```python
from build123d import *

# Parameters (mm, degrees)
RESSALTO_EXTRUS_O1_DEPTH = 0.3


with BuildPart() as part:
    # Esboço1 → Ressalto-extrusão1 (new body, symmetric)
    with BuildSketch(Plane.XY):
        with BuildLine():
            Line((17.891752756, 0.197947805), (17.891752756, -0.002052195))
            Line((17.891752756, -0.002052195), (17.091752756, -0.002052195))
            ThreePointArc((17.091752756, -0.002052195), (16.996884427, 0.013342816), (16.911752756, 0.057947805))
            Line((16.911752756, 0.057947805), (16.038199366, 0.968756691))
            ThreePointArc((16.038199366, 0.968756691), (16.005773821, 0.990473944), (15.967488688, 0.99804386))
            Line((15.967488688, 0.99804386), (12.407488688, 0.99))
            Line((12.407488688, 0.99), (10.557971552, 1.813458083))
            ThreePointArc((10.557971552, 1.813458083), (10.373577052, 1.832838725), (10.213007112, 1.740133627))
            Line((10.213007112, 1.740133627), (9.099531826, 0.503494039))
            Line((9.099531826, 0.503494039), (8.95090286, 0.637320161))
            Line((8.95090286, 0.637320161), (10.064378147, 1.873959748))
            ThreePointArc((10.064378147, 1.873959748), (10.331994714, 2.028468246), (10.639318881, 1.996167174))
            Line((10.639318881, 1.996167174), (12.45, 1.19))
            Line((12.45, 1.19), (15.967488688, 1.197947805))
            ThreePointArc((15.967488688, 1.197947805), (16.082345327, 1.175236263), (16.179620722, 1.11007984))
            Line((16.179620722, 1.11007984), (17.029007121, 0.256846352))
            ThreePointArc((17.029007121, 0.256846352), (17.094002269, 0.213258484), (17.170747658, 0.197947805))
            Line((17.170747658, 0.197947805), (17.891752756, 0.197947805))
        make_face()
    extrude(amount=RESSALTO_EXTRUS_O1_DEPTH, both=True)


solid = part.part
```
Source: CAD feature listing. Evaluate the final solid. Frame: model axes, mm. Give positions to 0.01 mm unless a question says otherwise; leave off trailing zeros. Loops run counter-clockwise (first coordinate to the right, second up) from the corner with the lowest first, then second, coordinate; pieces in that order, holes last. Notation, with made-up numbers: M -11.75,-12 L 21.25,-12 A27 cw 21.25,15 Z; hole C -9.75,-1.75 d1. An arc over 180 degrees is marked long. Put each result on its own line as item: value.
Q1. Line query: probe 1 along Y at (x, z) = (17.25, 0); probe 2 along Y at (x, z) = (15.5, -0.15); probe 3 along X at (y, z) = (0.95, -0.05). Output: solid intervals per line, ascending. Write a range as [from, to].
Response values:
probe 1: y = [0, 0.2]
probe 2: y = [1, 1.2]
probe 3: x = [9.23, 9.5], [16.06, 16.34]
Q2. Section C-C (y = 0.8). Return the cut outline in (x, z).
Response values:
outline: M 9.1,-0.3 L 9.37,-0.3 L 9.37,0.3 L 9.1,0.3 Z; M 16.2,-0.3 L 16.49,-0.3 L 16.49,0.3 L 16.2,0.3 Z
Q3. Pin query (flat end, axial travel): P1, Ø1, axis at x = 13, y = 1.5, coming from the -Z side. Return the tip coordinate at first contact, or that it passes through.
Response values:
P1: stops at z = -0.3
Q4. Section A-A (y = 1.3). Return the cut outline in (x, z).
Response values:
outline: M 9.55,-0.3 L 9.82,-0.3 L 9.82,0.3 L 9.55,0.3 Z; M 11.71,-0.3 L 12.2,-0.3 L 12.2,0.3 L 11.71,0.3 Z
Q5. Section B-B (z = 0.05). Return the cut outline in (x, y), and give its area (3 significant figures).
Response values:
outline: M 8.95,0.64 L 9.1,0.5 L 10.21,1.74 A0.3 cw 10.56,1.81 L 12.41,0.99 L 15.97,1 A0.1 cw 16.04,0.97 L 16.91,0.06 A0.3 ccw 17.09,0 L 17.89,0 L 17.89,0.2 L 17.17,0.2 A0.2 cw 17.03,0.26 L 16.18,1.11 A0.3 ccw 15.97,1.2 L 12.45,1.19 L 10.64,2 A0.5 ccw 10.06,1.87 Z
area: 2.02 mm²
Q6. Section D-D (x = 12). Return the cut outline in (y, z), and give its area (3 significant figures).
Response values:
outline: M 1.17,-0.3 L 1.39,-0.3 L 1.39,0.3 L 1.17,0.3 Z
area: 0.131 mm²
Q7. Mould query, pull axis X, two halves, no side actions, for faces 1 (the flat face through (9.5, 1.25, 0)), 2 (the flat face through (16.48, 0.51, 0)), 3 (the flat face through (16.6, 0.69, 0)). Classes: released by +X, released by -X, zero draft, split by the parting line, or undercut.
Response values:
face 1: released by -X
face 2: undercut
face 3: released by +X
